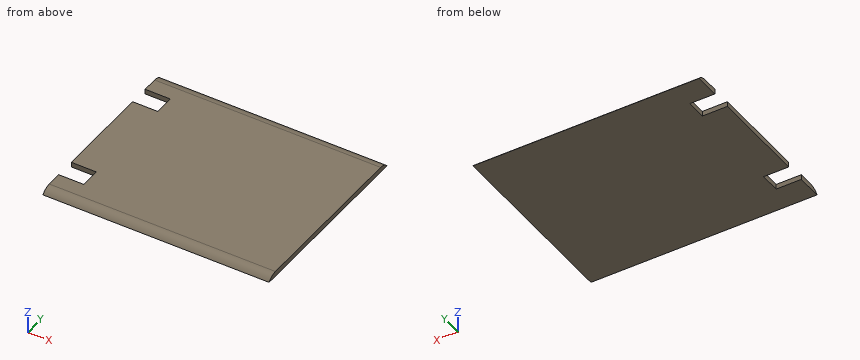
from build123d import *

# Parameters (mm, degrees)
F1_DEPTH    = 2
F2_T1_DEPTH = 110


# Not quite as in the source:
# - a fillet or chamfer that OpenCascade refuses, or shapes differently, is made with other operations: its cross-section is extruded or revolved along the edge and cut away or added


with BuildPart() as f1:
    # F0 (on Top) → F1 (new body)
    with BuildSketch(Plane.XY):
        Polygon((45, 27.5), (-35, 27.5), (-35, 19.5), (-45, 19.5), (-45, -19.5), (-35, -19.5), (-35, -27.5), (45, -27.5), align=None)
        Polygon((-45, 37.5), (-45, 27.5), (-35, 27.5), (45, 27.5), (45, 37.5), align=None)
        Polygon((45, -37.5), (45, -27.5), (-35, -27.5), (-45, -27.5), (-45, -37.5), align=None)
    extrude(amount=F1_DEPTH)

    # F2: fillet of radius 5 on 2 edges, made by hand

    # F2_s2 → F2_t1 (cut)
    with BuildSketch(Plane.YZ.offset(-55)):
        with BuildLine():
            ThreePointArc((37.5, 0), (35.7360679775, 1.472135955), (33.5, 2))
            Line((33.5, 2), (37.5, 2))
            Line((37.5, 2), (37.5, 0))
        make_face()
        with BuildLine():
            ThreePointArc((-37.5, 0), (-35.7360679775, 1.472135955), (-33.5, 2))
            Line((-33.5, 2), (-37.5, 2))
            Line((-37.5, 2), (-37.5, 0))
        make_face()
    extrude(amount=F2_T1_DEPTH, mode=Mode.SUBTRACT)


solid = f1.part
Design review of the part built by this model. Coordinates are the model's own, in mm. Coordinates: 2 decimals unless noted, no trailing zeros. Loops run counter-clockwise (first coordinate to the right, second up) from the corner with the lowest first, then second, coordinate; pieces in that order, holes last. Notation, with made-up numbers: (-39, 82) - (18, 82) arc R25 cw to (18, 96) - close; hole circle Ø10 at (38, -8). An arc over 180 degrees is marked (long way). Use CSV: the item, a comma, the result in double quotes. Start each with the question number.
1. Add section B-B on x = -8. Give the boundary of the cut face in (y, z), plus the area to 3 significant figures.
2. To check wall thickness, follow probe 1 along X at (y, z) = (26, 1.75); probe 2 along Y at (x, z) = (1, 1.45); probe 3 along Y at (x, z) = (-18, 1.6). State the ranges of each line that lie inside material, in increasing order.
3. Clearance check with flat-ended pins moving along their axes: pin 1 (1 mm diameter, centred on y = 23, z = 1.5, fed in from -X); pin 2 (4 mm diameter, centred on x = 27.5, y = -18, fed in from -Z); pin 3 (1 mm diameter, centred on x = -42, z = 1, fed in from -Y). State where each tip first meets the part, or that it passes through.
4. Add section A-A on z = 1.7. Give the boundary of the cut face in (x, y), plus the area to 3 significant figures.
Resolved:
1,outline,"(-37.5, 0) - (37.5, 0) arc R5 ccw to (33.5, 2) - (-33.5, 2) arc R5 ccw to start"
1,area,"145 mm2"
2,probe 1,"-35 to 45"
2,probe 2,"-35.78 to 35.78"
2,probe 3,"-35.46 to 35.46"
3,pin 1,"x = -35"
3,pin 2,"z = 0"
3,pin 3,"y = -37.07"
4,outline,"(-45, -35.21) - (45, -35.21) - (45, 35.21) - (-45, 35.21) - (-45, 27.5) - (-35, 27.5) - (-35, 19.5) - (-45, 19.5) - (-45, -19.5) - (-35, -19.5) - (-35, -27.5) - (-45, -27.5) - close"
4,area,"6,180 mm2"
